Part model, mm, in its own coordinate system. A direction names the side the tool comes from. Round coordinates to 2 decimals unless told otherwise and drop trailing zeros. Loops run counter-clockwise (first coordinate to the right, second up) from the corner with the lowest first, then second, coordinate; pieces in that order, holes last. Notation, with made-up numbers: M 61,20 L 65,20 A17 ccw 65,49 Z; hole C 27,11.25 d11. An arc over 180 degrees is marked long. Put each result on its own line as item: value. Start each with the question number.
```python
from build123d import *

# Parameters (mm, degrees)
SKETCH_1_W      = 5
SKETCH_1_H      = 3.5
EXTRUDE_1_DEPTH = 3.5
FILLET_1_R      = 5


with BuildPart() as part:
    # По траектории1: sweep along a path in Эскиз2
    with BuildLine(Plane(origin=(0, 6.25, 0), x_dir=(-1, 0, 0), z_dir=(0, -1, 0))) as sweep_1_path:
        Line((30.926565187, 15.32695004), (30.926565187, -11.67304996))
        ThreePointArc((30.926565187, -11.67304996), (30.633671968, -12.380156741), (29.926565187, -12.67304996))
        Line((29.926565187, -12.67304996), (2.926565187, -12.67304996))
        ThreePointArc((2.926565187, -12.67304996), (2.219458406, -12.380156741), (1.926565187, -11.67304996))
        Line((1.926565187, -11.67304996), (1.926565187, 15.32695004))
        ThreePointArc((1.926565187, 15.32695004), (2.219458406, 16.034056821), (2.926565187, 16.32695004))
        Line((2.926565187, 16.32695004), (29.926565187, 16.32695004))
        ThreePointArc((29.926565187, 16.32695004), (30.633671968, 16.034056821), (30.926565187, 15.32695004))
    # Эскиз1 → По траектории1 (sweep)
    with BuildSketch(Plane(origin=(0.073434813, 0, -1.82695004), x_dir=(1, 0, 0), z_dir=(0, 0, -1))):
        with Locations((-33.5, -8)):
            Rectangle(SKETCH_1_W, SKETCH_1_H)
    sweep(path=sweep_1_path.line)

    # Эскиз3 → Бобышка-Вытянуть1 (add)
    with BuildSketch(Plane(origin=(0, 9.75, 0), x_dir=(1, 0, 0), z_dir=(0, 1, 0))):
        with BuildLine():
            Line((-38.926565187, 9.32695004), (-35.926565187, 9.32695004))
            Line((-35.926565187, 9.32695004), (-35.926565187, -5.67304996))
            Line((-35.926565187, -5.67304996), (-38.926565187, -5.67304996))
            ThreePointArc((-38.926565187, -5.67304996), (-46.426565187, 1.82695004), (-38.926565187, 9.32695004))
        make_face()
    extrude(amount=-EXTRUDE_1_DEPTH)

    # Скругление1
    fillet_1_edges = [part.edges().sort_by_distance(p)[0] for p in [
        (-35.926565187, 8, -9.32695004),
        (-35.926565187, 8, 5.67304996),
    ]]
    fillet(fillet_1_edges, radius=FILLET_1_R)


solid = part.part
```
1. Cut at C-C, the plane z = -18. Give the cut face in (x, y).
2. Drop flat-ended pins along their axis: pin 1 (1.8 mm diameter, centred on y = 7, z = -6.5, fed in from -X); pin 2 (0.6 mm diameter, centred on y = 7.5, z = 11, fed in from -X). Give the stop position or say it passes through.
3. Wall check: L1, parallel to Z at x = -25.5, y = 7.1; L2, parallel to X at y = 7.45, z = 11.5; L3, parallel to X at y = 9.1, z = 8.5. Give the ranges that are in metal, low to high.
4. Mould opens along Z. For faces 4 (the cylindrical face through (-46.425, 8.024, -1.679)), 5 (the cylindrical face through (-30.63, 7.98, -16.04)), 6 (the flat face through (-35.927, 8, 11)) say: released by +Z, released by -Z, zero draft, split by the parting line, or undercut.
5. Cut at B-B, the plane z = -1. Give the cut face in (x, y).
6. Cut at A-A, the plane x = -16. Give the cut face in (y, z), and give its area (3 significant figures).
7. Which spindle directions (+Z, -Z, +X, -X, +Y, -Y) get a long thin tool onto all of the face, cutting with end or side? Do faces 1 (the cylindrical face through (-30.641, 7.976, 12.372)), 2 (the cylindrical face through (1.362, 8.024, -19.523)), 3 (the flat face through (-35.927, 8, -15)). Say none if no direction does.
8. Cut at D-D, the plane x = 0.5. Give the cut face in (y, z).
Results list:
1. outline: M -35.3,6.25 L 2.45,6.25 L 2.45,9.75 L -35.3,9.75 Z
2. pin 1: stops at x = -45.41
2. pin 2: stops at x = -35.93
3. L1: z = -21.33 to -16.33, 12.67 to 17.67
3. L2: x = -35.93 to -30.93, -1.93 to 3.07
3. L3: x = -36.35 to -30.93, -1.93 to 3.07
4. face 4: split by the parting line
4. face 5: undercut
4. face 6: zero draft
5. outline: M -46.38,6.25 L -30.93,6.25 L -30.93,9.75 L -46.38,9.75 Z; M -1.93,6.25 L 3.07,6.25 L 3.07,9.75 L -1.93,9.75 Z
6. outline: M 6.25,-21.33 L 9.75,-21.33 L 9.75,-16.33 L 6.25,-16.33 Z; M 6.25,12.67 L 9.75,12.67 L 9.75,17.67 L 6.25,17.67 Z
6. area: 35.0 mm^2
7. face 1: +Y, -Y
7. face 2: -Z, +X, +Y, -Y
7. face 3: -Z, -X, +Y, -Y
8. outline: M 6.25,-20.25 L 9.75,-20.25 L 9.75,16.6 L 6.25,16.6 Z
